Check sheet for the modelled part. Datum: model origin and axes. Units: mm. Face numbers are marked on the shaded views. A direction names the side the tool comes from. Give positions to 0.01 mm unless a question says otherwise; leave off trailing zeros. Loops run counter-clockwise (first coordinate to the right, second up) from the corner with the lowest first, then second, coordinate; pieces in that order, holes last.
Autodesk Inventor part; units mm, degrees
ref_plane "YZ Plane" through (0, 0, 0) normal (1, 0, 0) x (0, 1, 0)
ref_plane "XZ Plane" through (0, 0, 0) normal (0, 1, 0) x (-1, 0, 0)
ref_plane "XY Plane" through (0, 0, 0) normal (0, 0, 1) x (1, 0, 0)
sketch "스케치1" plane through (0, 0, 0) normal (1, 0, 0) x (0, 1, 0)
  line L0 (-5, 5) -> (5, 5)
  line L1 (5, 5) -> (5, -5)
  line L2 (5, -5) -> (-5, -5)
  line L3 (-5, -5) -> (-5, 5)
  line L4 (-5, 5) -> (5, -5) construction
  line L5 (5, 5) -> (-5, -5) construction
  point P0 (0, 0)
  dimension "d0" = 10
  dimension "d1" = 10
extrude "돌출1" add sketch "스케치1" along normal blind 3
sketch "스케치2" plane through (0, 5, 5) normal (0, 1, 0) x (1, 0, 0)
  line L0 (0, 10) -> (0, 0)
  line L1 (0, 0) -> (3, 0)
  line L2 (3, 10) -> (3, 0)
  line L3 (0, 10) -> (3, 10)
  line L4 (0, 0) -> (10, 0)
  line L5 (10, 0) -> (10, 10)
  line L6 (10, 10) -> (0, 10)
  line L7 (0, 10) -> (0, 0)
  point P0 (0, 5)
  dimension "d4" = 10
  dimension "d5" = 10
extrude "돌출2" add sketch "스케치2" along normal blind 3
sketch "스케치3" plane through (0, -5, 5) normal (0, 0, 1) x (1, 0, 0)
  line L0 (0, 0) -> (0, 13)
  line L1 (0, 0) -> (3, 0)
  line L2 (3, 10) -> (3, 0)
  line L3 (3, 10) -> (10, 10)
  line L4 (10, 10) -> (10, 13)
  line L5 (0, 13) -> (10, 13)
  line L6 (0, 13) -> (10, 13)
  line L7 (10, 13) -> (10, 0)
  line L8 (10, 0) -> (0, 0)
  line L9 (0, 0) -> (0, 13)
  point P0 (0, 5)
extrude "돌출3" add sketch "스케치3" along normal blind 3
sketch "스케치4" plane through (3, 0, 0) normal (1, 0, 0) x (0, 0, -1)
  circle A0 centre (0, 0) radius 1.25
  dimension "d10" = 2.5
extrude "돌출4" cut sketch "스케치4" against normal blind 3
sketch "스케치5" plane through (0, 5, 5) normal (0, -1, 0) x (1, 0, 0)
  line L0 (3, -10) -> (3, 0)
  line L1 (10, -10) -> (3, -10)
  line L2 (10, 0) -> (10, -10)
  line L3 (3, 0) -> (10, 0)
  line L4 (10, 0) -> (10, -10)
  line L5 (10, -5) -> (6.5, -5)
  line L6 (6.5, -5) -> (6.5, -10)
  circle A0 centre (6.5, -5) radius 1.25
  point P0 (0, -5)
  dimension "d13" = 2.5
extrude "돌출5" cut sketch "스케치5" against normal blind 3 contours A0 L5 L6 | L6 L5 A0
sketch "스케치6" plane through (0, -5, 5) normal (0, 0, -1) x (-1, 0, 0)
  line L0 (-3, 10) -> (-10, 10)
  line L1 (-10, 0) -> (-10, 10)
  line L2 (-3, 0) -> (-10, 0)
  line L3 (-3, 10) -> (-3, 0)
  line L4 (-3, 0) -> (-10, 0)
  line L5 (-6.5, 0) -> (-6.5, 5)
  line L6 (-6.5, 5) -> (-3, 5)
  circle A0 centre (-6.5, 5) radius 1.25
  point P0 (0, 5)
  dimension "d16" = 2.5
extrude "돌출6" cut sketch "스케치6" against normal blind 3 contours A0 L5 L6 | L6 L5 A0
properties part number "64" material "LCP 플라스틱"
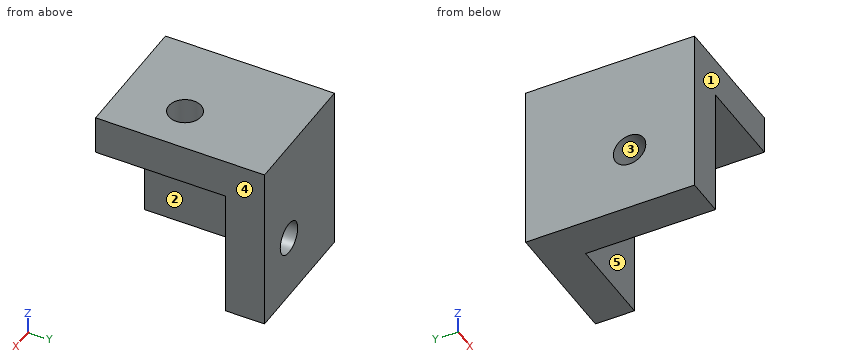
(1) Access from +Z, -Z, +X, -X, +Y, -Y to the whole of each face (thin tool, end or side, straight path). Record for the marked faces 4 and 5.
(2) Section check C-C on y = -3. Record the boundary of the cut face in (x, z).
(3) Section check D-D on x = 2.75. Record the boundary of the cut face in (y, z).
(4) Section check A-A on y = 0. Record the boundary of the cut face in (x, z), plus the area to 3 significant figures.
(5) Section check B-B on x = 6.5. Record the boundary of the cut face in (y, z), plus the area to 3 significant figures.
(6) Material ranges on line 1 (X direction, y = 6.95, z = 0); line 2 (Z direction, x = 6.5, y = 5.9), recorded low to high.
(7) Release check for a two-part mould opening along Y. For the marked faces 1, 2 and 3 record: pulls with the +Y half, pulls with the -Y half, needs draft (parallel to the pull), parting line crosses it, or undercut.
(8) Gauge pin test, flat ends, axial feed: pin 1 Ø5 at (y, z) = (-2, -1.5) entering from +X; pin 2 Ø5 at (x, z) = (7.5, -1) entering from -Y; pin 3 Ø5.5 at (x, y) = (6.5, 2) entering from -Z; pin 4 Ø2 at (x, y) = (6.5, 0) entering from -Z. Record the tip position at first contact, or that the pin passes through.
Computed values:
1. face 4: +Z, -Z, +X, +Y, -Y
1. face 5: -Z, +X, -Y
2. outline: (0, -5) - (3, -5) - (3, 5) - (10, 5) - (10, 8) - (0, 8) - close
3. outline: (-5, -5) - (8, -5) - (8, 8) - (-5, 8) - close; hole circle Ø2.5 at (0, 0)
4. outline: (0, -5) - (3, -5) - (3, -1.25) - (0, -1.25) - close; (0, 1.25) - (3, 1.25) - (3, 5) - (5.25, 5) - (5.25, 8) - (0, 8) - close; (7.75, 5) - (10, 5) - (10, 8) - (7.75, 8) - close
4. area: 45.0 mm2
5. outline: (-5, 5) - (-1.25, 5) - (-1.25, 8) - (-5, 8) - close; (1.25, 5) - (5, 5) - (5, 1.25) - (8, 1.25) - (8, 8) - (1.25, 8) - close; (5, -5) - (8, -5) - (8, -1.25) - (5, -1.25) - close
5. area: 54.0 mm2
6. line 1: x = 0 to 5.25, 7.75 to 10
6. line 2: z = -5 to -1.25, 1.25 to 8
7. face 1: pulls with the -Y half
7. face 2: needs draft
7. face 3: undercut
8. pin 1: stops at x = 3
8. pin 2: stops at y = 5
8. pin 3: stops at z = 5
8. pin 4: passes through
